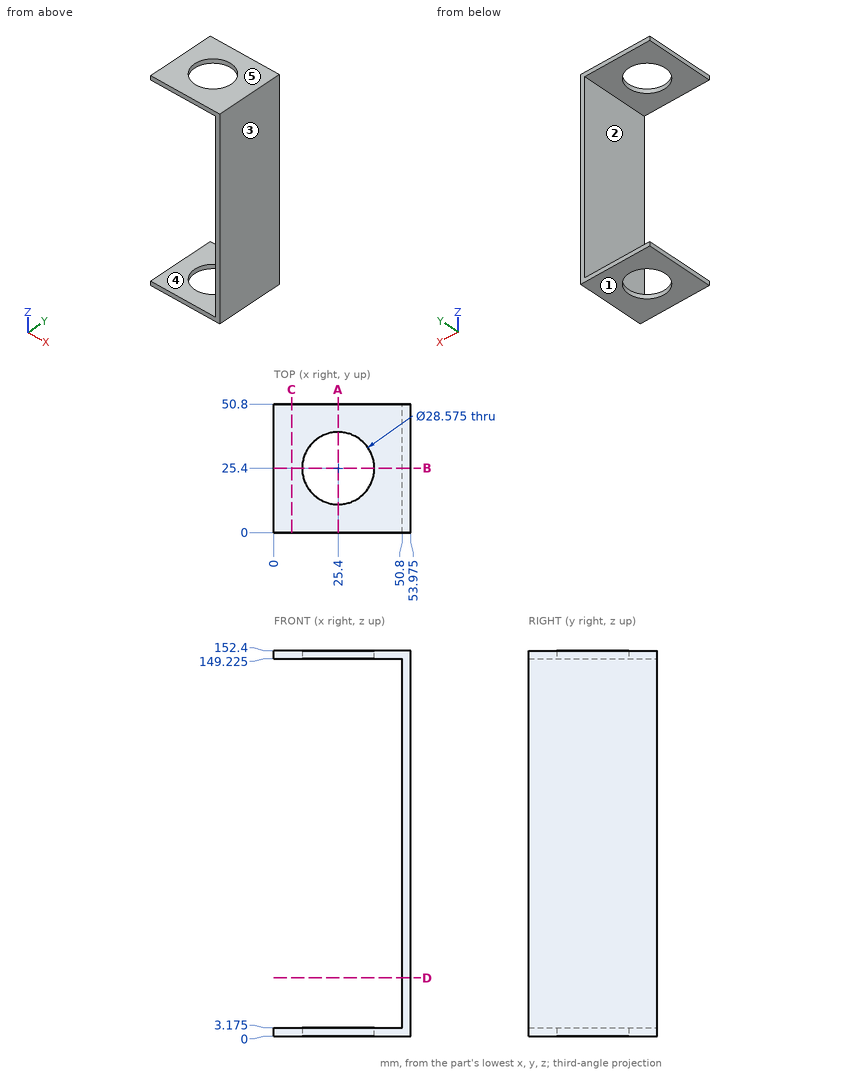
Print and shaded views of the part. All mm, measured from the part's lowest x, y and z. A direction names the side the tool comes from. Give positions to 0.01 mm unless a question says otherwise; leave off trailing zeros. Write each loop counter-clockwise with the first axis right and the second up, starting at its lowest first coordinate (ties: lowest second). Pieces come first, ordered by that corner, then holes. Notation, with made-up numbers: M 86.5,-4.75 L 95.5,-4.75 A17 ccw 95.5,2.25 Z; hole C -26.75,89.25 d11. An arc over 180 degrees is marked long. Use a Markdown table: item, result.
1) Cut at D-D (z = 23). List the corners of the cut face in (x, y) (3 decimals).
Responses:
| item | result |
|---|---|
| outline | M 50.8,0 L 53.975,0 L 53.975,50.8 L 50.8,50.8 Z |
2) Pull direction Z, two halves, no side cores. Call the marked faces 3, 4 and 5: +Z half, -Z half, draft (parallel to the pull), parting line (faces both ways), or undercut.
Responses:
| item | result |
|---|---|
| face 3 | draft |
| face 4 | undercut |
| face 5 | +Z half |
3) Cut at A-A (x = 25.4). List the corners of the cut face in (y, z) (1 decimal).
Responses:
| item | result |
|---|---|
| outline | M 0,0 L 11.1,0 L 11.1,3.2 L 0,3.2 Z; M 0,149.2 L 11.1,149.2 L 11.1,152.4 L 0,152.4 Z; M 39.7,0 L 50.8,0 L 50.8,3.2 L 39.7,3.2 Z; M 39.7,149.2 L 50.8,149.2 L 50.8,152.4 L 39.7,152.4 Z |
4) Tool access for the marked faces 1 and 2: list every direction of +Z, -Z, +X, -X, +Y, -Y with a clear straight run to the whole face (end or side of a thin tool).
Responses:
| item | result |
|---|---|
| face 1 | -Z, +X, -X, +Y, -Y |
| face 2 | -X, +Y, -Y |
5) Cut at C-C (x = 7). List the corners of the cut face in (y, z) (3 decimals).
Responses:
| item | result |
|---|---|
| outline | M 0,0 L 50.8,0 L 50.8,3.175 L 0,3.175 Z; M 0,149.225 L 50.8,149.225 L 50.8,152.4 L 0,152.4 Z |
6) Pin check, flat tip, straight feed: pin 1 (3 mm diameter, centred on y = 33.5, z = 71.5, fed in from -X). Stop position of the tip, or through.
Responses:
| item | result |
|---|---|
| pin 1 | stops at x = 50.8 |
7) Cut at B-B (y = 25.4). List the corners of the cut face in (x, z) (1 decimal), and give its area (3 significant figures).
Responses:
| item | result |
|---|---|
| outline | M 0,0 L 11.1,0 L 11.1,3.2 L 0,3.2 Z; M 0,149.2 L 11.1,149.2 L 11.1,152.4 L 0,152.4 Z; M 39.7,0 L 54,0 L 54,152.4 L 39.7,152.4 L 39.7,149.2 L 50.8,149.2 L 50.8,3.2 L 39.7,3.2 Z |
| area | 625 mm2 |
8) Drill centre lines: line 1 (Z direction, x = 10, y = 26.5) (3 decimals); line 2 (Y direction, x = 25, z = 1); line 3 (X direction, y = 25, z = 151) (3 decimals). Where is each one in solid material? Low to high. Write a range as from..to.
Responses:
| item | result |
|---|---|
| line 1 | z = 0..3.175, 149.225..152.4 |
| line 2 | y = 0..11.12, 39.68..50.8 |
| line 3 | x = 0..11.118, 39.682..53.975 |
